CAD build for the part. Positions are in the model's coordinates, mm. Face numbers are marked on the shaded views. Coordinates: 2 decimals unless noted, no trailing zeros. Loops run counter-clockwise (first coordinate to the right, second up) from the corner with the lowest first, then second, coordinate; pieces in that order, holes last. Notation, with made-up numbers: (-6, -16) -> (53, -16) arc R21 ccw to (53, 5) -> close; hole circle Ø8 at (70.25, 0.5). An arc over 180 degrees is marked (long way). Write each question's results on one line, items separated by ' | '.
Autodesk Fusion 360 part; units mm, degrees
sketch "Sketch1" plane through (0, 0, 0) normal (0, 1, 0) x (1, 0, 0)
  line L0 (5, 12.5) -> (-5, 12.5)
  line L1 (-5, 12.5) -> (-5, -12.5)
  line L2 (-5, -12.5) -> (5, -12.5)
  line L3 (5, -12.5) -> (5, 12.5)
  line L4 (5, 12.5) -> (-5, -12.5) construction
  line L5 (-5, 12.5) -> (5, -12.5) construction
  arc A0 (5, 12.5) -> (-5, 12.5) centre (0, 12.5) ccw
  line L6 (-5, 0) -> (5, 0) construction
  circle A1 centre (0, 12.5) radius 1.5
  arc A2 (-5, -12.5) -> (5, -12.5) centre (0, -12.5) ccw
  circle A3 centre (0, -12.5) radius 1.5
  dimension "d1" = 10
  dimension "d2" = 25
  dimension "d3" = 3
extrude "Extrude1" add sketch "Sketch1" along normal blind 3 contours L0 L1 L2 L3 A1 A3 | L0 A0 A1 | L2 A2 A3 | L2 A3 | L2 A3
sketch "Boceto2" plane through (0, 3, 0) normal (0, 1, 0) x (-1, 0, 0)
  circle A0 centre (0, -12.5) radius 1.5
  arc A1 (5, 12.5) -> (-5, 12.5) centre (0, 12.5) ccw
  line L0 (-5, 12.5) -> (-5, -12.5)
  arc A2 (-5, -12.5) -> (5, -12.5) centre (0, -12.5) ccw
  line L1 (5, -12.5) -> (5, 12.5)
  circle A3 centre (0, 12.5) radius 2.63
  line L2 (0, 9.87) -> (0, 15.13) construction
  line L3 (0, 10.1418) -> (0.322, 9.8898)
  line L4 (0, 10.1418) -> (-0.322, 9.8898)
  line L5 (0.7287, 10.2572) -> (1.1128, 10.117)
  line L6 (0.7287, 10.2572) -> (0.5004, 9.918)
  line L7 (1.3861, 10.5922) -> (1.7947, 10.5776)
  line L8 (1.3861, 10.5922) -> (1.2737, 10.199)
  line L9 (1.9078, 11.1139) -> (2.301, 11.2263)
  line L10 (1.9078, 11.1139) -> (1.9224, 10.7053)
  line L11 (2.2428, 11.7713) -> (2.582, 11.9996)
  line L12 (2.2428, 11.7713) -> (2.383, 11.3872)
  line L13 (2.3582, 12.5) -> (2.6102, 12.822)
  line L14 (2.3582, 12.5) -> (2.6102, 12.178)
  line L15 (2.2428, 13.2287) -> (2.383, 13.6128)
  line L16 (2.2428, 13.2287) -> (2.582, 13.0004)
  line L17 (1.9078, 13.8861) -> (1.9224, 14.2947)
  line L18 (1.9078, 13.8861) -> (2.301, 13.7737)
  line L19 (1.3861, 14.4078) -> (1.2737, 14.801)
  line L20 (1.3861, 14.4078) -> (1.7947, 14.4224)
  line L21 (0.7287, 14.7428) -> (0.5004, 15.082)
  line L22 (0.7287, 14.7428) -> (1.1128, 14.883)
  line L23 (0, 14.8582) -> (-0.322, 15.1102)
  line L24 (0, 14.8582) -> (0.322, 15.1102)
  line L25 (-0.7287, 14.7428) -> (-1.1128, 14.883)
  line L26 (-0.7287, 14.7428) -> (-0.5004, 15.082)
  line L27 (-1.3861, 14.4078) -> (-1.7947, 14.4224)
  line L28 (-1.3861, 14.4078) -> (-1.2737, 14.801)
  line L29 (-1.9078, 13.8861) -> (-2.301, 13.7737)
  line L30 (-1.9078, 13.8861) -> (-1.9224, 14.2947)
  line L31 (-2.2428, 13.2287) -> (-2.582, 13.0004)
  line L32 (-2.2428, 13.2287) -> (-2.383, 13.6128)
  line L33 (-2.3582, 12.5) -> (-2.6102, 12.178)
  line L34 (-2.3582, 12.5) -> (-2.6102, 12.822)
  line L35 (-2.2428, 11.7713) -> (-2.383, 11.3872)
  line L36 (-2.2428, 11.7713) -> (-2.582, 11.9996)
  line L37 (-1.9078, 11.1139) -> (-1.9224, 10.7053)
  line L38 (-1.9078, 11.1139) -> (-2.301, 11.2263)
  line L39 (-1.3861, 10.5922) -> (-1.2737, 10.199)
  line L40 (-1.3861, 10.5922) -> (-1.7947, 10.5776)
  line L41 (-0.7287, 10.2572) -> (-0.5004, 9.918)
  line L42 (-0.7287, 10.2572) -> (-1.1128, 10.117)
  dimension "d6" = 5.26
  dimension "d7" = 0.252
  dimension "d8" = 0.322
  dimension "d10" = 360
extrude "Extruir2" cut sketch "Boceto2" against normal blind 2.6 contours A3 L3 L4 L5 L6 L7 L8 L9 L10 L11 L12 L13 L14 L15 L16 L17 L18 L19 L20 L21 L22 L23 L24 L25 L26 L27 L28 L29 L30 L31 L32 L33 L34 L35 L36 L37 L38 L39 L40 L41 L42
sketch "Boceto3" plane through (0, 0.4, 0) normal (0, 1, 0) x (-1, 0, 0)
  arc A0 (-0.5004, 9.918) -> (-0.322, 9.8898) centre (0, 12.5) ccw
  line L0 (-0.322, 9.8898) -> (0, 10.1418)
  line L1 (0, 10.1418) -> (0.322, 9.8898)
  arc A1 (0.322, 9.8898) -> (0.5004, 9.918) centre (0, 12.5) ccw
  line L2 (0.5004, 9.918) -> (0.7287, 10.2572)
  line L3 (0.7287, 10.2572) -> (1.1128, 10.117)
  arc A2 (1.1128, 10.117) -> (1.2737, 10.199) centre (0, 12.5) ccw
  line L4 (1.2737, 10.199) -> (1.3861, 10.5922)
  line L5 (1.3861, 10.5922) -> (1.7947, 10.5776)
  arc A3 (1.7947, 10.5776) -> (1.9224, 10.7053) centre (0, 12.5) ccw
  line L6 (1.9224, 10.7053) -> (1.9078, 11.1139)
  line L7 (1.9078, 11.1139) -> (2.301, 11.2263)
  arc A4 (2.301, 11.2263) -> (2.383, 11.3872) centre (0, 12.5) ccw
  line L8 (2.383, 11.3872) -> (2.2428, 11.7713)
  line L9 (2.2428, 11.7713) -> (2.582, 11.9996)
  arc A5 (2.582, 11.9996) -> (2.6102, 12.178) centre (0, 12.5) ccw
  line L10 (2.6102, 12.178) -> (2.3582, 12.5)
  line L11 (2.3582, 12.5) -> (2.6102, 12.822)
  arc A6 (2.6102, 12.822) -> (2.582, 13.0004) centre (0, 12.5) ccw
  line L12 (2.582, 13.0004) -> (2.2428, 13.2287)
  line L13 (2.2428, 13.2287) -> (2.383, 13.6128)
  arc A7 (2.383, 13.6128) -> (2.301, 13.7737) centre (0, 12.5) ccw
  line L14 (2.301, 13.7737) -> (1.9078, 13.8861)
  line L15 (1.9078, 13.8861) -> (1.9224, 14.2947)
  arc A8 (1.9224, 14.2947) -> (1.7947, 14.4224) centre (0, 12.5) ccw
  line L16 (1.7947, 14.4224) -> (1.3861, 14.4078)
  line L17 (1.3861, 14.4078) -> (1.2737, 14.801)
  arc A9 (1.2737, 14.801) -> (1.1128, 14.883) centre (0, 12.5) ccw
  line L18 (1.1128, 14.883) -> (0.7287, 14.7428)
  line L19 (0.7287, 14.7428) -> (0.5004, 15.082)
  arc A10 (0.5004, 15.082) -> (0.322, 15.1102) centre (0, 12.5) ccw
  line L20 (0.322, 15.1102) -> (0, 14.8582)
  line L21 (0, 14.8582) -> (-0.322, 15.1102)
  arc A11 (-0.322, 15.1102) -> (-0.5004, 15.082) centre (0, 12.5) ccw
  line L22 (-0.5004, 15.082) -> (-0.7287, 14.7428)
  line L23 (-0.7287, 14.7428) -> (-1.1128, 14.883)
  arc A12 (-1.1128, 14.883) -> (-1.2737, 14.801) centre (0, 12.5) ccw
  line L24 (-1.2737, 14.801) -> (-1.3861, 14.4078)
  line L25 (-1.3861, 14.4078) -> (-1.7947, 14.4224)
  arc A13 (-1.7947, 14.4224) -> (-1.9224, 14.2947) centre (0, 12.5) ccw
  line L26 (-1.9224, 14.2947) -> (-1.9078, 13.8861)
  line L27 (-1.9078, 13.8861) -> (-2.301, 13.7737)
  arc A14 (-2.301, 13.7737) -> (-2.383, 13.6128) centre (0, 12.5) ccw
  line L28 (-2.383, 13.6128) -> (-2.2428, 13.2287)
  line L29 (-2.2428, 13.2287) -> (-2.582, 13.0004)
  arc A15 (-2.582, 13.0004) -> (-2.6102, 12.822) centre (0, 12.5) ccw
  line L30 (-2.6102, 12.822) -> (-2.3582, 12.5)
  line L31 (-2.3582, 12.5) -> (-2.6102, 12.178)
  arc A16 (-2.6102, 12.178) -> (-2.582, 11.9996) centre (0, 12.5) ccw
  line L32 (-2.582, 11.9996) -> (-2.2428, 11.7713)
  line L33 (-2.2428, 11.7713) -> (-2.383, 11.3872)
  arc A17 (-2.383, 11.3872) -> (-2.301, 11.2263) centre (0, 12.5) ccw
  line L34 (-2.301, 11.2263) -> (-1.9078, 11.1139)
  line L35 (-1.9078, 11.1139) -> (-1.9224, 10.7053)
  arc A18 (-1.9224, 10.7053) -> (-1.7947, 10.5776) centre (0, 12.5) ccw
  line L36 (-1.7947, 10.5776) -> (-1.3861, 10.5922)
  line L37 (-1.3861, 10.5922) -> (-1.2737, 10.199)
  arc A19 (-1.2737, 10.199) -> (-1.1128, 10.117) centre (0, 12.5) ccw
  line L38 (-1.1128, 10.117) -> (-0.7287, 10.2572)
  line L39 (-0.7287, 10.2572) -> (-0.5004, 9.918)
  circle A20 centre (0, 12.5) radius 1.375
  dimension "d13" = 2.75
extrude "Extruir3" cut sketch "Boceto3" against normal blind 0.5 contours A20
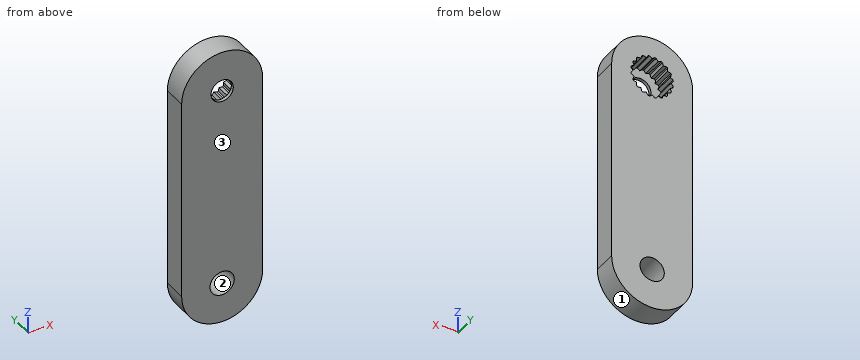
Q1. Cut at B-B on x = 3.5. Write the cut outline in (y, z), and give its area (3 significant figures).
Results are:
outline: (0, -16.07) -> (3, -16.07) -> (3, 16.07) -> (0, 16.07) -> close | area: 96.4 mm^2
Q2. Cut at A-A on y = 1.8. Give the number of separate pieces and of enclosed holes in the cut face, and give its area (3 significant figures).
Results are:
separate pieces: 1 | enclosed holes: 2 | area: 302 mm^2
Q3. Drop flat-ended pins along their axis: pin 1 (4.5 mm diameter, centred on x = 0, z = 12.5, fed in from +Y); pin 2 (4 mm diameter, centred on x = -1, z = 12.5, fed in from +Y); pin 3 (1 mm diameter, centred on x = -3, y = 2, fed in from -Z). Give the stop position or say it passes through.
Results are:
pin 1: y = 0.4 | pin 2: y = 3 | pin 3: z = -16.83
Q4. Wall check: L1, parallel to Z at x = 0, y = 0.1 (3 decimals); L2, parallel to X at y = 1.55, z = -12.5; L3, parallel to Z at x = -1.25, y = 1.65. Give the ranges that are in metal, low to high. Write a range as from..to.
Results are:
L1: -17.5..-14, -11..11.125, 13.875..17.5 | L2: -5..-1.5, 1.5..5 | L3: -17.34..-13.33, -11.67..10.19, 14.81..17.34
Q5. Pull direction X, two halves, no side cores. Call the marked faces 1, 2 and 3: +X half, -X half, draft (parallel to the pull), parting line (faces both ways), or undercut.
Results are:
face 1: parting line | face 2: undercut | face 3: draft
